Read the model definition and answer for the solid it produces. Units are mm, in the model's axes. Face numbers are marked on the shaded views. A direction names the side the tool comes from. Give positions to 0.01 mm unless a question says otherwise; leave off trailing zeros. Order: outer loops, then holes, each group sorted by start corner. A loop starts at its lowest first (then second) coordinate and runs counter-clockwise, first axis right, second up.
```python
from build123d import *

# Parameters (mm, degrees)
F0_R     = 16
F1_DEPTH = 70
F3_DEPTH = 30.001
F4_W     = 30
F4_H     = 12
F5_DEPTH = 120.001


with BuildPart() as f1:
    # F0 (on Front) → F1 (new body)
    with BuildSketch(Plane.XZ):
        with BuildLine():
            Line((-60, -35), (60, -35))
            Line((60, -35), (60, 5))
            ThreePointArc((60, 5), (30, 35), (0, 5))
            Line((0, 5), (0, -5))
            Line((0, -5), (-60, -5))
            Line((-60, -5), (-60, -35))
        make_face()
        with Locations((30, 5)):
            Circle(F0_R, mode=Mode.SUBTRACT)
    extrude(amount=F1_DEPTH)

    # F2 (on face) → F3 (cut, through all)
    with BuildSketch(Plane.XY.offset(-5)):
        with BuildLine():
            Line((-45, -58), (-29, -58))
            ThreePointArc((-29, -58), (-25.464466, -56.535534), (-24, -53))
            Line((-24, -53), (-24, -17))
            ThreePointArc((-24, -17), (-25.464466, -13.464466), (-29, -12))
            Line((-29, -12), (-45, -12))
            ThreePointArc((-45, -12), (-48.535534, -13.464466), (-50, -17))
            Line((-50, -17), (-50, -53))
            ThreePointArc((-50, -53), (-48.535534, -56.535534), (-45, -58))
        make_face()
    extrude(amount=-F3_DEPTH, mode=Mode.SUBTRACT)

    # F4 (on face) → F5 (cut, through all)
    with BuildSketch(Plane(origin=(-60, 0, 0), x_dir=(0, -1, 0), z_dir=(-1, 0, 0))):
        with Locations((35, -29)):
            Rectangle(F4_W, F4_H)
    extrude(amount=-F5_DEPTH, mode=Mode.SUBTRACT)


solid = f1.part
```
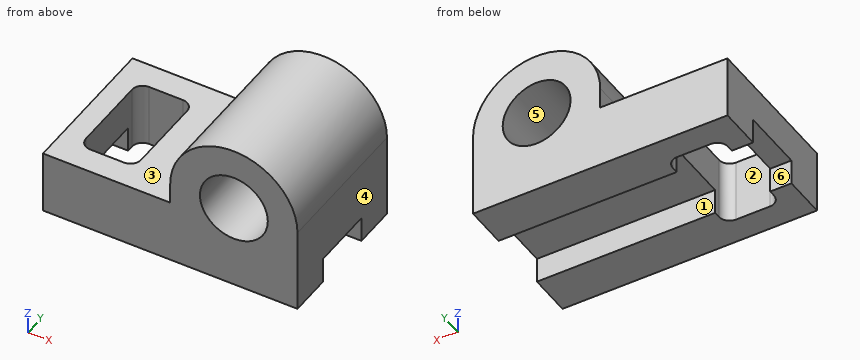
1) Consider L1, parallel to X at y = -38.5, z = -15; L2, parallel to Z at x = 30, y = -26; L3, parallel to X at y = -44, z = -6. Determine where each line is inside the solid, lowest interval first.
Final values:
L1: x = -60 to -50, -24 to 60
L2: z = -23 to -11, 21 to 35
L3: x = -60 to -50, -24 to 18.38, 41.62 to 60
2) A tool of negligible diameter and unlimited length cuts with its end or side. For the marked faces 1, 2 and 3, from which of +Z, -Z, +X, -X, +Y, -Y can it reach the whole face along a straight path? Write none if from no direction.
Final values:
face 1: -Z, +X, -X
face 2: +Z, -Z
face 3: +Z, -X, +Y, -Y
3) The part is cut by section C-C on z = 12.5. Determine the outline of the cut face in (x, y).
Final values:
outline: (0.95, -70) - (15.87, -70) - (15.87, 0) - (0.95, 0) - close; (44.13, -70) - (59.05, -70) - (59.05, 0) - (44.13, 0) - close
4) The part is cut by section A-A on y = -46.5. Determine the outline of the cut face in (x, z), and give its area (3 significant figures).
Final values:
outline: (-60, -23) - (-50, -23) - (-50, -5) - (-60, -5) - close; (-24, -23) - (60, -23) - (60, 5) arc R30 ccw to (0, 5) - (0, -5) - (-24, -5) - close; hole circle Ø32 at (30, 5)
area: 2,900 mm2
5) For a pull along X with two mould halves and no side action, classify the marked faces 4, 5 and 6 as released by +X, released by -X, zero draft, split by the parting line, or undercut.
Final values:
face 4: released by +X
face 5: undercut
face 6: zero draft
6) Given pin 1 (12 mm diameter, centred on x = 43, y = -52, fed in from +Z); pin 2 (4 mm diameter, centred on x = -31.5, y = -9, fed in from +Z); pin 3 (2 mm diameter, centred on y = -44, z = 10, fed in from +X); pin 4 (12 mm diameter, centred on y = -42, z = -4, fed in from -X), each flat-ended and moving along its own axis, determine where each tip first touches the part or whether it passes through.
Final values:
pin 1: stops at z = 34.17
pin 2: stops at z = -5
pin 3: stops at x = 59.73
pin 4: stops at x = -60
7) The part is cut by section B-B on x = 30. Determine the outline of the cut face in (y, z).
Final values:
outline: (-70, -35) - (-50, -35) - (-50, -23) - (-20, -23) - (-20, -35) - (0, -35) - (0, -11) - (-70, -11) - close; (-70, 21) - (0, 21) - (0, 35) - (-70, 35) - close
8) The part is cut by section D-D on x = -12. Determine the outline of the cut face in (y, z).
Final values:
outline: (-70, -35) - (-50, -35) - (-50, -23) - (-20, -23) - (-20, -35) - (0, -35) - (0, -5) - (-70, -5) - close
